from build123d import *

# Parameters (mm, degrees)
SKETCH2_R           = 3.175
SKETCH2_R_2         = 5.9817
CUT_EXTRUDE1_DEPTH  = 76.878222264
CUT_EXTRUDE3_DEPTH  = 10.6934
SKETCH5_W           = 19.304
SKETCH5_H           = 37.8079
BOSS_EXTRUDE1_DEPTH = 12.4587
SKETCH6_R           = 17.5641
BOSS_EXTRUDE2_DEPTH = 25.6032
SKETCH7_R           = 9.03605
BOSS_EXTRUDE3_DEPTH = 64.4271
CUT_EXTRUDE2_DEPTH  = 1.524


with BuildPart() as part:
    # Sketch1 → Revolve1 (revolve)
    with BuildSketch(Plane.XY, mode=Mode.PRIVATE) as revolve1_sk:
        Polygon((0, 0), (-46.101, 0), (-48.895, 31.242), (-45.0572124, 31.242), (-43.495525408, 13.7795), (0, 13.7795), align=None)
    revolve(revolve1_sk.sketch.rotate(Axis((0, 0, 0), (0, 1, 0)), 270), axis=Axis((0, 0, 0), (0, 1, 0)))

    # Sketch2 → Cut-Extrude1 (cut, through all)
    with BuildSketch(Plane.XZ):
        with Locations(Location((16.891, 0, 0), (0, 0, 270))):
            Circle(SKETCH2_R)
        with Locations(Location((-32.4993, 0, 0), (0, 0, 270))):
            Circle(SKETCH2_R_2)
    extrude(amount=-CUT_EXTRUDE1_DEPTH, mode=Mode.SUBTRACT)

    # Sketch4 → Cut-Extrude3 (cut)
    with BuildSketch(Plane(origin=(0, 13.7795, 0), x_dir=(1, 0, 0), z_dir=(0, 1, 0))):
        with BuildLine():
            Line((-32.372904727, -10.50925), (-42.206828772, -10.50925))
            ThreePointArc((-42.206828772, -10.50925), (-43.495497734, -0.049065379), (-42.23043138, 10.414))
            Line((-42.23043138, 10.414), (-32.403671088, 10.414))
            ThreePointArc((-32.403671088, 10.414), (34.035963204, 0.050047806), (-32.372904727, -10.50925))
        make_face()
    extrude(amount=-CUT_EXTRUDE3_DEPTH, mode=Mode.SUBTRACT)

    # Sketch5 → Boss-Extrude1 (add)
    with BuildSketch(Plane.XZ):
        Rectangle(SKETCH5_W, SKETCH5_H)
    extrude(amount=BOSS_EXTRUDE1_DEPTH)

    # Sketch6 → Boss-Extrude2 (add)
    with BuildSketch(Plane(origin=(0, 3.0861, 0), x_dir=(1, 0, 0), z_dir=(0, 1, 0))):
        with Locations(Location((0, 0, 0), (0, 0, 10.335443893))):
            Circle(SKETCH6_R)
    extrude(amount=BOSS_EXTRUDE2_DEPTH)

    # Sketch7 → Boss-Extrude3 (add)
    with BuildSketch(Plane(origin=(0, 28.6893, 0), x_dir=(1, 0, 0), z_dir=(0, 1, 0))):
        with Locations(Location((0, 0, 0), (0, 0, 270))):
            Circle(SKETCH7_R)
    extrude(amount=BOSS_EXTRUDE3_DEPTH)

    # Sketch3 → Cut-Extrude2 (cut)
    with BuildSketch(Plane(origin=(0, 3.0861, 0), x_dir=(1, 0, 0), z_dir=(0, 1, 0))):
        Polygon((22.44725, -3.207902433), (22.44725, 3.207902433), (16.891, 6.415804866), (11.33475, 3.207902433), (11.33475, -3.207902433), (16.891, -6.415804866), align=None)
    extrude(amount=-CUT_EXTRUDE2_DEPTH, mode=Mode.SUBTRACT)


solid = part.part
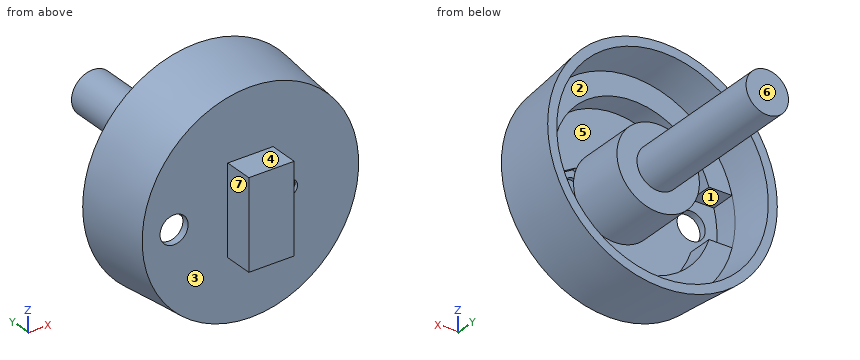
CAD build for the part. Positions are in the model's coordinates, mm. Face numbers are marked on the shaded views. A direction names the side the tool comes from. Round coordinates to 2 decimals unless told otherwise and drop trailing zeros. Order: outer loops, then holes, each group sorted by start corner. A loop starts at its lowest first (then second) coordinate and runs counter-clockwise, first axis right, second up. Notation, with made-up numbers: (80.25, -38.5) -> (119.25, -38.5) arc R17 cw to (119.25, -30.5) -> close; hole circle Ø5 at (-25, -0.75). An arc over 180 degrees is marked (long way). Write item = value, one per line. Start each with the question number.
(1) Cut at A-A, the plane y = 7.5. List the corners of the cut face in (x, z).
(2) Probe line 1 (X direction, y = 1, z = 0); line 2 (Z direction, x = 8.5, y = 26.5); line 3 (X direction, y = 14.5, z = 0). List the from-to ranges inside material, lowest first. Write a range as [from, to].
(3) Cut at D-D, the plane y = 71.5. List the corners of the cut face in (x, z).
(4) Pull direction Z, two halves, no side cores. Call the marked faces 1, 2, 3 and 4: released by +Z, released by -Z, zero draft, split by the parting line, or undercut.
(5) Which spindle directions (+Z, -Z, +X, -X, +Y, -Y) get a long thin tool onto all of the face, cutting with end or side? Do the marked faces 5, 6 and 7. Say none if no direction does.
(6) Cut at B-B, the plane x = 0. List the corners of the cut face in (y, z) (1 decimal).
(7) Cut at C-C, the plane z = 0. State how many separate pieces and enclosed holes the cut face has, then the cut area to 3 significant figures.
(8) Pin check, flat tips, straight feed: P1, Ø2, axis at x = -4, y = 52.5, coming from the -Z side; P2, Ø12, axis at x = 19, z = -1.5, coming from the +Y side; P3, Ø8, axis at x = 35.5, z = 0.5, coming from the +Y side. Stop position of each tip, or through.
Model answer:
q1.outline = circle Ø93.54 at (0, 0); circle Ø35.13 at (0, 0); hole (-42.23, -10.41) -> (-32.4, -10.41) arc R34.04 ccw (long way) to (-32.37, 10.51) -> (-42.21, 10.51) arc R43.5 ccw to start
q2.line_1 = [-46.19, -38.48], [-26.52, 13.72], [20.07, 46.19]
q2.line_2 = [-47.72, -43.82], [-15.37, 15.37], [43.82, 47.72]
q2.line_3 = [-47.4, -43.56], [-17.56, 17.56], [43.56, 47.4]
q3.outline = circle Ø18.07 at (0, 0)
q4.face_1 = undercut
q4.face_2 = undercut
q4.face_3 = zero draft
q4.face_4 = released by +Z
q5.face_5 = +Y
q5.face_6 = +Z, -Z, +X, -X, +Y
q5.face_7 = +Z, -Z, -X, -Y
q6.outline = (-12.5, -18.9) -> (0, -18.9) -> (0, -46.1) -> (31.2, -48.9) -> (31.2, -45.1) -> (13.8, -43.5) -> (13.8, -34) -> (3.1, -34) -> (3.1, -17.6) -> (28.7, -17.6) -> (28.7, -9) -> (93.1, -9) -> (93.1, 9) -> (28.7, 9) -> (28.7, 17.6) -> (3.1, 17.6) -> (3.1, 34) -> (13.8, 34) -> (13.8, 43.5) -> (31.2, 45.1) -> (31.2, 48.9) -> (0, 46.1) -> (0, 18.9) -> (-12.5, 18.9) -> close
q7.separate_pieces = 3
q7.enclosed_holes = 0
q7.area = 2,830 mm2
q8.P1 = -8.52
q8.P2 = 28.69
q8.P3 = 13.78
